For this review, use the dimensioned drawing (mm, ordinates from the lowest corner) and the shaded views. Give positions to 0.01 mm unless a question says otherwise; leave off trailing zeros. Use a Markdown table: item, result. Add a question column.
(1) Add section A-A, the plane x = 78.55. State how many separate pieces and enclosed holes the cut face has, then the cut area to 3 significant figures.
(2) For probe 1 along X at (y, z) = (1.9, 4); probe 2 along Z at (x, y) = (78.55, 1.3); probe 3 along Z at (x, y) = (71, 0.5), list the stretches that pass through material, from the lowest coordinate up.
(3) Insertion check: pin 1 Ø1.4 at (x, z) = (70.775, 11.575) entering from -Y. The pin has a flat end and moves straight along its axis. Give the tip position at first contact, or say it passes through.
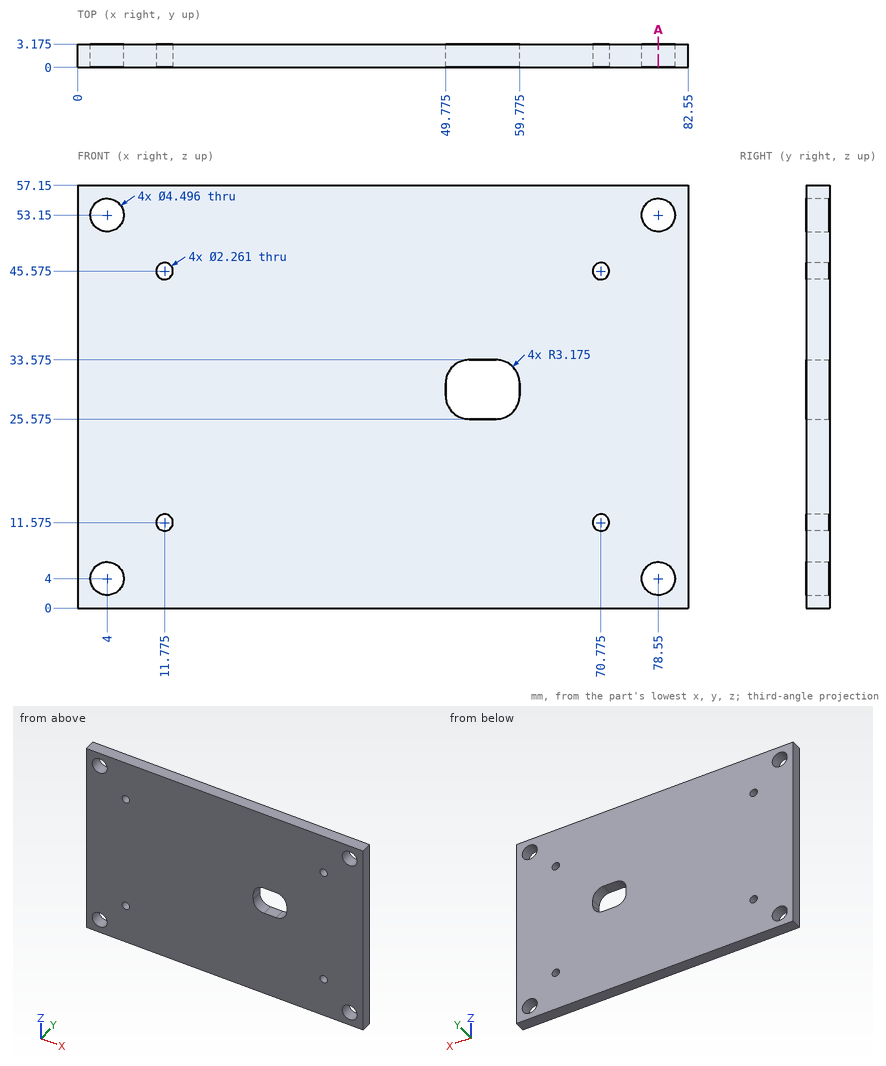
Established:
| question | item | result |
|---|---|---|
| 1 | separate pieces | 3 |
| 1 | enclosed holes | 0 |
| 1 | area | 153 mm^2 |
| 2 | probe 1 | 0 to 1.75, 6.25 to 76.3, 80.8 to 82.55 |
| 2 | probe 2 | 0 to 1.75, 6.25 to 50.9, 55.4 to 57.15 |
| 2 | probe 3 | 0 to 10.47, 12.68 to 44.47, 46.68 to 57.15 |
| 3 | pin 1 | through |
